Here's how the part is built. I have some questions about the finished solid (model axes, mm). A direction names the side the tool comes from. Round coordinates to 2 decimals unless told otherwise and drop trailing zeros. Write each loop counter-clockwise with the first axis right and the second up, starting at its lowest first coordinate (ties: lowest second). Pieces come first, ordered by that corner, then holes. Notation, with made-up numbers: (-3, 35) -> (28, 35) arc R21 cw to (28, 66) -> close; hole circle Ø10 at (56.25, -30.75). An arc over 180 degrees is marked (long way). Answer in a Markdown table with one row per item. Add a question column.
from build123d import *

# Parameters (mm, degrees)
CYLINDER004_R     = 2
CYLINDER004_DEPTH = 2.3
ARRAY_X_COUNT     = 2
ARRAY_X_PITCH     = 10
CYLINDER003_R     = 2.5
CYLINDER003_DEPTH = 10
ARRAY001_X_COUNT  = 11
ARRAY001_X_PITCH  = 10
BOX001_W          = 150
BOX001_H          = 13
BOX001_DEPTH      = 1.5
FILLET001_R       = 4.5


with BuildPart() as button_clone:
    # Sketch → Revolve (revolve)
    with BuildSketch(Plane.XZ):
        with BuildLine():
            Line((-2.2, 0), (0, 0))
            Line((0, 0), (0, 3.513454))
            add(Edge.make_bspline(
                [(0, 3.513454), (-0.678463, 3.195757), (-0.989147, 2.937398), (-1.619509, 2.257916), (-2.069526, 1.674454)],
                knots=[0, 0, 0, 0, 0.5, 1, 1, 1, 1], degree=3))
            add(Edge.make_bspline(
                [(-2.069526, 1.674454), (-2.787947, 1.236244), (-3.158335, 0.790309), (-3.182894, 0.331863), (-2.2, 0)],
                knots=[0, 0, 0, 0, 0.5, 1, 1, 1, 1], degree=3))
        make_face()
    revolve(axis=Axis((0, 0, 0), (0, 0, 1)))


with BuildPart() as button_clone_1:
    # Body001 placement: moved
    add(button_clone.part.moved(Location((0, 0, 2.3))))


with BuildPart() as button_array:
    # Cylinder004 → Cylinder004 (new body)
    with BuildSketch(Plane.XY):
        Circle(CYLINDER004_R)
    extrude(amount=CYLINDER004_DEPTH)

    # Fusion002: union button clone
    add(button_clone_1.part)

    # Array X: button_array ×2


with BuildPart() as button_array_1:
    add(button_array.part)
    with Locations(*[(i * ARRAY_X_PITCH, 0, 0) for i in range(1, ARRAY_X_COUNT)]):
        add(button_array.part)


with BuildPart() as button_array_2:
    # Array placement: moved
    add(button_array_1.part.moved(Location((4, 6.5, 1.5))))


with BuildPart() as button_hole_array:
    # Cylinder003 → Cylinder003 (new body)
    with BuildSketch(Plane.XY):
        Circle(CYLINDER003_R)
    extrude(amount=CYLINDER003_DEPTH)

    # Array001 X: button hole array ×11


with BuildPart() as button_hole_array_1:
    add(button_hole_array.part)
    with Locations(*[(i * ARRAY001_X_PITCH, 0, 0) for i in range(1, ARRAY001_X_COUNT)]):
        add(button_hole_array.part)


with BuildPart() as button_hole_array_2:
    # Array001 placement: moved
    add(button_hole_array_1.part.moved(Location((44, 6.5, 0))))


with BuildPart() as strap_union:
    # Box001 → Box001 (new body)
    with BuildSketch(Plane.XY):
        with Locations((75, 6.5)):
            Rectangle(BOX001_W, BOX001_H)
    extrude(amount=BOX001_DEPTH)

    # Fillet001
    fillet001_edges = [strap_union.edges().sort_by_distance(p)[0] for p in [
        (0, 0, 0.75),
        (0, 13, 0.75),
        (150, 0, 0.75),
        (150, 13, 0.75),
    ]]
    fillet(fillet001_edges, radius=FILLET001_R)

    # Cut002: cut button hole array
    add(button_hole_array_2.part, mode=Mode.SUBTRACT)

    # Fusion001: union button_array
    add(button_array_2.part)


solid = strap_union.part
Item 1: If we section it at A-A on x = 64: Please give me the cut outline in (y, z).
Item 2: I need wall thicknesses on line 1 along Y through (x, z) = (124, 0.75); line 2 along Z through (x, y) = (117, 12); line 3 along X through (y, z) = (7.25, 4). Which ranges of each line are inside material? Lowest first, please. Write a range as from..to.
Item 3: If we section it at B-B on x = 133: Please give me the cut outline in (y, z).
Item 4: If we section it at C-C on x = 36: Please give me the cut outline in (y, z), then the cut area to 3 significant figures.
Item 5: On a 3-axis mill with a long thin cutter (end or side, diameter ignored), from which of +Z, -Z, +X, -X, +Y, -Y can I reach the whole of each face in a straight line? I mean faces 4 (the flat face through (74, 9.5, 0)), 5 (the cylindrical face through (12.526, 7.852, 2.634)). Say none if no direction works.
Item 6: If we mould it in two halves opening along Y, with no side actions, what happens to faces 1 (the cylindrical face through (148.647, 1.283, 0.76)), 2 (the cylindrical face through (116.385, 7.251, 0.74)), 3 (the cylindrical face through (2.526, 7.852, 2.634))? For each: pulls with the +Y half, pulls with the -Y half, needs draft (parallel to the pull), parting line crosses it, or undercut.
Item 7: For P1, Ø6.5, axis at x = 74, y = 6.5, coming from the +Z side, with a flat end and sliding along its axis, tell me the tip position at first contact or that it passes through.
Results list:
| question | item | result |
|---|---|---|
| 1 | outline | (0, 0) -> (4, 0) -> (4, 1.5) -> (0, 1.5) -> close; (9, 0) -> (13, 0) -> (13, 1.5) -> (9, 1.5) -> close |
| 2 | line 1 | 0..4, 9..13 |
| 2 | line 2 | 0..1.5 |
| 2 | line 3 | 1.4..6.6, 11.4..16.6 |
| 3 | outline | (0, 0) -> (4.21, 0) -> (4.21, 1.5) -> (0, 1.5) -> close; (8.79, 0) -> (13, 0) -> (13, 1.5) -> (8.79, 1.5) -> close |
| 4 | outline | (0, 0) -> (13, 0) -> (13, 1.5) -> (0, 1.5) -> close |
| 4 | area | 19.5 mm² |
| 5 | face 4 | -Z, +X, -X, +Y, -Y |
| 5 | face 5 | none |
| 6 | face 1 | pulls with the -Y half |
| 6 | face 2 | undercut |
| 6 | face 3 | parting line crosses it |
| 7 | P1 | z = 1.5 |
